The listing builds one solid part. Answer for the finished solid, in the listing's coordinates (mm). Coordinates: 2 decimals unless noted, no trailing zeros. Order: outer loops, then holes, each group sorted by start corner. A loop starts at its lowest first (then second) coordinate and runs counter-clockwise, first axis right, second up. Notation, with made-up numbers: (-18.75, 28.25) -> (0.25, 28.25) arc R31 cw to (0.25, 60.25) -> close; hole circle Ø6 at (-33.75, 66). An arc over 180 degrees is marked (long way). Write item = value, one per line. Start each with the question number.
Solid Edge part; units mm, degrees
sketch "Sketch1" plane through (9.0161, -6.1697, 0) normal (0, 0, 1) x (1, 0, 0)
  line L0 (-10.0161, 5.1697) -> (-10.0161, -111.8903)
  arc A0 (-10.0161, -111.8903) -> (-9.0161, -112.8903) centre (-9.0161, -111.8903) ccw
  line L1 (-9.0161, -112.8903) -> (47.0839, -112.8903)
  arc A1 (47.0839, -112.8903) -> (48.0839, -111.8903) centre (47.0839, -111.8903) ccw
  line L2 (48.0839, -111.8903) -> (48.0839, -111.0328)
  arc A2 (48.0839, -111.0328) -> (49.0839, -110.0328) centre (49.0839, -111.0328) cw
  line L3 (49.0839, -110.0328) -> (66.1339, -110.0328)
  arc A3 (66.1339, -110.0328) -> (67.1339, -109.0328) centre (66.1339, -109.0328) ccw
  line L4 (67.1339, -109.0328) -> (67.1339, -108.1753)
  arc A4 (67.1339, -108.1753) -> (68.1339, -107.1753) centre (68.1339, -108.1753) cw
  line L5 (68.1339, -107.1753) -> (71.8467, -107.1753)
  arc A5 (71.8467, -107.1753) -> (72.3467, -107.3093) centre (71.8467, -108.1753) cw
  line L6 (72.3467, -107.3093) -> (135.2985, -143.6546)
  arc A6 (135.2985, -143.6546) -> (136.6646, -143.2885) centre (135.7985, -142.7885) ccw
  line L7 (136.6646, -143.2885) -> (162.1493, -99.1476)
  arc A7 (162.1493, -99.1476) -> (161.7833, -97.7816) centre (161.2833, -98.6476) ccw
  line L8 (161.7833, -97.7816) -> (150.9766, -91.5423)
  arc A8 (150.9766, -91.5423) -> (150.4766, -90.6763) centre (151.4766, -90.6763) cw
  line L9 (150.4766, -90.6763) -> (150.4766, 5.1695)
  arc A9 (150.4766, 5.1695) -> (149.4766, 6.1695) centre (149.4766, 5.1695) ccw
  line L10 (149.4766, 6.1695) -> (106.2339, 6.1695)
  arc A10 (106.2339, 6.1695) -> (105.2339, 7.1695) centre (106.2339, 7.1695) cw
  line L11 (105.2339, 7.1695) -> (105.2339, 8.0272)
  arc A11 (105.2339, 8.0272) -> (104.2339, 9.0272) centre (104.2339, 8.0272) ccw
  line L12 (104.2339, 9.0272) -> (87.1839, 9.0272)
  arc A12 (87.1839, 9.0272) -> (86.1839, 10.0272) centre (87.1839, 10.0272) cw
  line L13 (86.1839, 10.0272) -> (86.1839, 10.8847)
  arc A13 (86.1839, 10.8847) -> (85.1839, 11.8847) centre (85.1839, 10.8847) ccw
  line L14 (85.1839, 11.8847) -> (48.1339, 11.8847)
  arc A14 (48.1339, 11.8847) -> (47.1339, 10.8847) centre (48.1339, 10.8847) ccw
  line L15 (47.1339, 10.8847) -> (47.1339, 10.0306)
  arc A15 (47.1339, 10.0306) -> (46.1339, 9.0306) centre (46.1339, 10.0306) cw
  line L16 (46.1339, 9.0306) -> (29.0839, 9.0306)
  arc A16 (29.0839, 9.0306) -> (28.0839, 8.0306) centre (29.0839, 8.0306) ccw
  line L17 (28.0839, 8.0306) -> (28.0839, 7.1697)
  arc A17 (28.0839, 7.1697) -> (27.0839, 6.1697) centre (27.0839, 7.1697) cw
  line L18 (27.0839, 6.1697) -> (-9.0161, 6.1697)
  arc A18 (-9.0161, 6.1697) -> (-10.0161, 5.1697) centre (-9.0161, 5.1697) ccw
extrude "Protrusion1" add sketch "Sketch1" against normal blind 3
properties material "ABS Plastic, high impact"
Item 1: For a pull along X with two mould halves and no side action, classify faces 1 (the flat face through (165.472, -100.875, -1.479)), 2 (the flat face through (84, -54, 0)) as pulls with the +X half, pulls with the -X half, needs draft (parallel to the pull), parting line crosses it, or undercut.
Item 2: Each of these flat-tipped pins is pushed along its axis until it touches: pin 1 (0.7 mm diameter, centred on y = -115, z = -2, fed in from +X); pin 2 (1.5 mm diameter, centred on y = -47.5, z = -2, fed in from +X); pin 3 (0.7 mm diameter, centred on y = -117.5, z = -1.5, fed in from +X). Where does it stop, or does it pass through?
Item 3: Section A-A, the plane y = -82 is taken. Give the vertices of the cut face in (x, z).
Item 4: Section B-B, the plane x = 71.5 is taken. Give the vertices of the cut face in (y, z) (1 decimal).
Item 5: Consider probe 1 along X at (y, z) = (-81.5, -0.8); probe 2 along Y at (x, z) = (68, -1.3) (1 decimal); probe 3 along Y at (x, z) = (18, -0.3). Determine where each line is inside the solid, lowest interval first.
A:
q1.face_1 = pulls with the +X half
q1.face_2 = needs draft
q2.pin_1 = 165.78
q2.pin_2 = 159.49
q2.pin_3 = 164.33
q3.outline = (-1, -3) -> (159.49, -3) -> (159.49, 0) -> (-1, 0) -> close
q4.outline = (-116.2, -3) -> (5.7, -3) -> (5.7, 0) -> (-116.2, 0) -> close
q5.probe_1 = -1 to 159.49
q5.probe_2 = -116.2 to 5.7
q5.probe_3 = -119.06 to 0
